from build123d import *

# Parameters (mm, degrees)
SKETCH1_R                                        = 19.25
SKETCH1_R_2                                      = 16.25
BOSS_EXTRUDE1_DEPTH                              = 5
BOSS_EXTRUDE2_DEPTH                              = 8
CBORE_FOR_1_4_SOCKET_HEAD_CAP_SCREW1_D           = 6.7564
CBORE_FOR_1_4_SOCKET_HEAD_CAP_SCREW1_CBORE_D     = 11.1125
CBORE_FOR_1_4_SOCKET_HEAD_CAP_SCREW1_CBORE_DEPTH = 6.35
FILLET1_R                                        = 10


with BuildPart() as part:
    # Sketch1 → Boss-Extrude1 (new body)
    with BuildSketch(Plane(origin=(0, 0, 0), x_dir=(1, 0, 0), z_dir=(0, 1, 0))):
        with Locations(Location((0, 0, 0), (0, 0, 270))):
            Circle(SKETCH1_R)
        with Locations(Location((0, 0, 0), (0, 0, 270))):
            Circle(SKETCH1_R_2, mode=Mode.SUBTRACT)
    extrude(amount=BOSS_EXTRUDE1_DEPTH)

    # Sketch2 → Boss-Extrude2 (add)
    with BuildSketch(Plane(origin=(0, 0, 0), x_dir=(1, 0, 0), z_dir=(0, 1, 0))):
        with BuildLine():
            Line((0, 27.35), (-39.35, 27.35))
            Line((-39.35, 27.35), (-39.35, -10.75))
            Line((-39.35, -10.75), (-15.968719423, -10.75))
            ThreePointArc((-15.968719423, -10.75), (-16.992645468, 9.045026258), (0, 19.25))
            Line((0, 19.25), (0, 27.35))
        make_face()
    extrude(amount=BOSS_EXTRUDE2_DEPTH)

    # CBORE for 1/4 Socket Head Cap Screw1 (through all)
    with Locations(Plane(origin=(0, 8, 0), x_dir=(1, 0, 0), z_dir=(0, 1, 0))):
        with Locations((-33, 21), (-33, -4.4)):
            CounterBoreHole(CBORE_FOR_1_4_SOCKET_HEAD_CAP_SCREW1_D / 2, CBORE_FOR_1_4_SOCKET_HEAD_CAP_SCREW1_CBORE_D / 2, CBORE_FOR_1_4_SOCKET_HEAD_CAP_SCREW1_CBORE_DEPTH)

    # Fillet1
    # the kernel refuses this fillet: 10 mm, written as the material it adds along each edge
    with BuildSketch(Plane(origin=(-15.968719423, 0, 10.75), x_dir=(0.6369824352168134, 0, 0.7708783154462564), z_dir=(0, 1, 0))) as fillet1_piece_1:
        with BuildLine():
            CenterArc((4.748847629, -9.951948419), FILLET1_R, 95.619084045, 44.81374241)
            Line((-2.959935525, -3.582124067), (0, 0))
            ThreePointArc((0, 0), (1.884851894, -0.092499293), (3.769703788, 0))
        make_face()
    extrude(amount=5)
    with BuildSketch(Plane(origin=(0, 0, -19.25), x_dir=(0.984823666621771, 0, 0.1735579029075042), z_dir=(0, 1, 0))) as fillet1_piece_2:
        with BuildLine():
            CenterArc((8.417558291, 9.848236666), FILLET1_R, 190.784553847, 69.220698266)
            Line((-1.405819014, 7.9770717), (0, 0))
            ThreePointArc((0, 0), (3.340989631, 0.292144418), (6.681979262, 0))
        make_face()
    extrude(amount=5)
    # the kernel refuses this fillet: 10 mm, written as the material it takes off along each edge
    with BuildSketch(Plane(origin=(0, 8, 0), x_dir=(-0.05010434447284765, 0, 0.998743988550092), z_dir=(0.998743988550092, 0, 0.05010434447284765))) as fillet1_2_piece_1:
        with BuildLine():
            CenterArc((26.391428429, 10), FILLET1_R, 224.427004001, 45.572995999)
            Line((26.391428429, 0), (19.25, 0))
            Line((19.25, 0), (19.25, 3))
        make_face()
    revolve(axis=Axis((0, 8, 0), (0, -1, 0)), revolution_arc=230.307970534, mode=Mode.SUBTRACT)


solid = part.part
Read the model definition and answer for the solid it produces. Units are mm, in the model's axes. A direction names the side the tool comes from. Give positions to 0.01 mm unless a question says otherwise; leave off trailing zeros. Write each loop counter-clockwise with the first axis right and the second up, starting at its lowest first coordinate (ties: lowest second). Pieces come first, ordered by that corner, then holes. Notation, with made-up numbers: (32, -22.5) - (57, -22.5) arc R18 cw to (57, -15.5) - close; hole circle Ø11 at (43.25, 81.5). An arc over 180 degrees is marked (long way). Use CSV: the item, a comma, the result in double quotes. Start each with the question number.
(1) Find section A-A (x = -33). Give the vertices of the cut face in (y, z), plus the area to 3 significant figures.
(2) Determine the mould class of faces 1 (the flat face through (-29, 1.65, -21)), 2 (the flat face through (-27, 8, -13)), 3 (the cylindrical face through (-16.753, 2.465, 11.526)) for opening direction Z: +Z half, -Z half, draft (parallel to the pull), parting line (faces both ways), or undercut.
(3) Find section C-C (z = 0). Give the vertices of the cut face in (x, y), plus the area to 3 significant figures.
(4) Find section B-B (y = 2.5). Give the vertices of the cut face in (x, z).
(5) For faces 4 (the flat face through (7, 5, -15)), 5 (the flat face through (0, 6, -24)), 6 (the flat face through (-18, 0, -7)), 7 (the cylindrical face through (-38.55, 4.87, 4.16)), 8 (the cylindrical face through (-36.222, 0.813, 3.385)), determine the directions among +Z, -Z, +X, -X, +Y, -Y from which every point of the face is accessible in a straight line to the end or side of a thin tool.
(6) Consider line 1 along Z through (x, y) = (-33, 1.05); line 2 along Z through (x, y) = (-29, 3.25); line 3 along X through (y, z) = (1.75, 1.5). Determine where each line is inside the solid, lowest interval first.
(7) Given P1, Ø6, axis at x = -33, z = -21, coming from the -Y side; P2, Ø4, axis at x = 4.5, y = 6, coming from the +Z side; P3, Ø9, axis at x = -35.5, z = 2, coming from the +Y side; P4, Ø3.5, axis at y = 6.5, z = -22, coming from the +X side, each flat-ended and moving along its own axis, determine where each tip first touches the part or whether it passes through.
Findings below:
1,outline,"(0, -27.35) - (8, -27.35) - (8, -26.56) - (1.65, -26.56) - (1.65, -24.38) - (0, -24.38) - close; (0, -17.62) - (1.65, -17.62) - (1.65, -15.44) - (8, -15.44) - (8, -1.16) - (1.65, -1.16) - (1.65, 1.02) - (0, 1.02) - close; (0, 7.78) - (1.65, 7.78) - (1.65, 9.96) - (8, 9.96) - (8, 10.75) - (0, 10.75) - close"
1,area,"141 mm2"
2,face 1,"undercut"
2,face 2,"draft"
2,face 3,"+Z half"
3,outline,"(-39.35, 0) - (-16.25, 0) - (-16.25, 5) - (-19.25, 5) arc R10 ccw to (-26.39, 8) - (-29.61, 8) - (-29.61, 1.65) - (-36.39, 1.65) - (-36.39, 8) - (-39.35, 8) - close; (16.25, 0) - (19.25, 0) - (19.25, 5) - (16.25, 5) - close"
3,area,"141 mm2"
4,outline,"(-39.35, -27.35) - (0, -27.35) arc R10 cw to (6.58, -18.09) arc R19.25 ccw (long way) to (-13.57, 13.66) arc R10 cw to (-20.62, 10.75) - (-39.35, 10.75) - close; hole circle Ø11.11 at (-33, -21); hole circle Ø11.11 at (-33, 4.4); hole circle Ø32.5 at (0, 0)"
5,face 4,"+X, +Y"
5,face 5,"+Z, -Z, +X, +Y"
5,face 6,"+Z, -Z, +X, -X, -Y"
5,face 7,"+Y"
5,face 8,"+Y, -Y"
6,line 1,"-27.35 to -24.38, -17.62 to 1.02, 7.78 to 10.75"
6,line 2,"-27.35 to -24.86, -17.14 to 0.54, 8.26 to 10.75"
6,line 3,"-39.35 to -37.74, -28.26 to -16.18, 16.18 to 19.19"
7,P1,"through"
7,P2,"z = 19.05"
7,P3,"y = 8"
7,P4,"x = 2.31"
